```python
from build123d import *

# Parameters (mm, degrees)
SKETCH1_W           = 101.6
SKETCH1_H           = 76.2
BOSS_EXTRUDE1_DEPTH = 38.1
SKETCH3_W           = 97.6
SKETCH3_H           = 72.2
CUT_EXTRUDE1_DEPTH  = 36.1
SKETCH7_R           = 2.54
CUT_EXTRUDE2_DEPTH  = 2
SKETCH9_R           = 4
CUT_EXTRUDE3_DEPTH  = 2
SKETCH11_R          = 3.175
CUT_EXTRUDE4_DEPTH  = 2
FILLET1_R           = 5
FILLET2_R           = 5
CUT_EXTRUDE5_DEPTH  = 1


with BuildPart() as part:
    # Sketch1 → Boss-Extrude1 (new body)
    with BuildSketch(Plane(origin=(0, 0, 0), x_dir=(1, 0, 0), z_dir=(0, 1, 0))):
        Rectangle(SKETCH1_W, SKETCH1_H)
    extrude(amount=BOSS_EXTRUDE1_DEPTH)

    # Sketch3 → Cut-Extrude1 (cut)
    with BuildSketch(Plane(origin=(0, 38.1, 0), x_dir=(1, 0, 0), z_dir=(0, 1, 0))):
        Rectangle(SKETCH3_W, SKETCH3_H)
    extrude(amount=-CUT_EXTRUDE1_DEPTH, mode=Mode.SUBTRACT)

    # Sketch7 → Cut-Extrude2 (cut)
    with BuildSketch(Plane(origin=(50.8, 0, 0), x_dir=(0, 0, -1), z_dir=(1, 0, 0))):
        with Locations((-19.05, 19.05)):
            Circle(SKETCH7_R)
        with Locations((19.05, 19.05)):
            Circle(SKETCH7_R)
    extrude(amount=-CUT_EXTRUDE2_DEPTH, mode=Mode.SUBTRACT)

    # Sketch9 → Cut-Extrude3 (cut)
    with BuildSketch(Plane.ZY.offset(50.8)):
        with Locations((0, 19.05)):
            Circle(SKETCH9_R)
    extrude(amount=-CUT_EXTRUDE3_DEPTH, mode=Mode.SUBTRACT)

    # Sketch11 → Cut-Extrude4 (cut)
    with BuildSketch(Plane.XY.offset(38.1)):
        with Locations((-34.127797524, 19.05)):
            Circle(SKETCH11_R)
    extrude(amount=-CUT_EXTRUDE4_DEPTH, mode=Mode.SUBTRACT)

    # Fillet1
    fillet1_edges = [part.edges().sort_by_distance(p)[0] for p in [
        (50.8, 19.05, 38.1),
        (-50.8, 19.05, 38.1),
        (-50.8, 19.05, -38.1),
        (50.8, 19.05, -38.1),
    ]]
    fillet(fillet1_edges, radius=FILLET1_R)

    # Fillet2
    fillet2_edges = [part.edges().sort_by_distance(p)[0] for p in [
        (48.8, 20.05, 36.1),
        (-48.8, 20.05, 36.1),
        (-48.8, 20.05, -36.1),
        (48.8, 20.05, -36.1),
    ]]
    fillet(fillet2_edges, radius=FILLET2_R)

    # Sketch12 → Cut-Extrude5 (cut)
    # profile 1 of 2: a face of its own
    with BuildSketch(Plane.XZ):
        Polygon((-16.893847177, 6.052120704), (-32.260033074, 6.052120704), (-24.77410559, 22.334171986), (-24.386134837, 22.334171986), align=None)
        Polygon((-19.09446817, 7.476800191), (-24.576940125, 19.395770544), (-30.056231992, 7.476800191), align=None, mode=Mode.SUBTRACT)
    # profile 2 of 2: a face of its own
    with BuildSketch(Plane.XZ):
        Polygon((-6.564920895, 6.052120704), (-15.774456151, 6.052120704), (-11.338233194, 14.110464053), (-15.774456151, 21.927120704), (-6.768446536, 21.927120704), (-6.768446536, 20.298915576), (-13.255826343, 20.298915576), (-9.61780551, 13.887857884), (-13.144523258, 7.476800191), (-6.564920895, 7.476800191), align=None)
    extrude(amount=-CUT_EXTRUDE5_DEPTH, mode=Mode.SUBTRACT)


solid = part.part
```
Read the model definition and answer for the solid it produces. Units are mm, in the model's axes. A direction names the side the tool comes from. Round coordinates to 2 decimals unless told otherwise and drop trailing zeros. Write each loop counter-clockwise with the first axis right and the second up, starting at its lowest first coordinate (ties: lowest second). Pieces come first, ordered by that corner, then holes. Notation, with made-up numbers: M 81,27.5 L 108,27.5 A34 ccw 108,66.5 Z; hole C 54,-34 d8. An arc over 180 degrees is marked long. One line per item, written item: value.
Q1. Find section A-A on z = 0. Write down the section's boundary in (x, y).
Data:
outline: M -50.8,0 L 50.8,0 L 50.8,38.1 L 48.8,38.1 L 48.8,2 L -48.8,2 L -48.8,15.05 L -50.8,15.05 Z; M -50.8,23.05 L -48.8,23.05 L -48.8,38.1 L -50.8,38.1 Z
Q2. Flat-ended cylindrical pins translate along their axes: pin 1 Ø10 at (x, z) = (7.5, -10.5) entering from +Y; pin 2 Ø4 at (y, z) = (20, -1.5) entering from -X; pin 3 Ø1.5 at (x, z) = (12, -25) entering from -Y. Find the tip coordinate at first contact, or state that the pin passes through.
Data:
pin 1: y = 2
pin 2: x = 48.8
pin 3: y = 0
Q3. Which of the six approach directions +Z, -Z, +X, -X, +Y, -Y give full straight-line access (tool end or side, diameter ignored) to faces 1 (the flat face through (-1, 19, 38.1)), 2 (the cylindrical face through (-49.37, 19.32, -36.6)), 3 (the cylindrical face through (-49.814, 15.145, -0.867)), 4 (the flat face through (-27.28, 0.49, 13.52)), 5 (the flat face through (-48.8, 24, 0))?
Data:
face 1: +Z, +X, -X, +Y, -Y
face 2: -Z, -X, +Y, -Y
face 3: -X
face 4: -Y
face 5: +Y
Q4. For a pull along Y with two mould halves and no side action, classify faces 6 (the flat face through (-1, 0, -1)), 7 (the flat face through (-11.356, 0.493, 10.727)), 8 (the cylindrical face through (49.81, 16.57, -18.5)) as +Y half, -Y half, draft (parallel to the pull), parting line (faces both ways), or undercut.
Data:
face 6: -Y half
face 7: draft
face 8: undercut
Q5. Find section B-B on y = 12. Write down the section's boundary in (x, z), plus the area to 3 significant figures.
Data:
outline: M -50.8,-33.1 A5 ccw -45.8,-38.1 L 45.8,-38.1 A5 ccw 50.8,-33.1 L 50.8,33.1 A5 ccw 45.8,38.1 L -45.8,38.1 A5 ccw -50.8,33.1 Z; hole M -48.8,-31.1 A5 ccw -43.8,-36.1 L 43.8,-36.1 A5 ccw 48.8,-31.1 L 48.8,31.1 A5 ccw 43.8,36.1 L -43.8,36.1 A5 ccw -48.8,31.1 Z
area: 695 mm2
Q6. Find section C-C on y = 19.05. Count the separate pieces of the cut face and the enclosed holes in it, plus the area to 3 significant figures.
Data:
separate pieces: 4
enclosed holes: 0
area: 646 mm2
Q7. Find section D-D on x = 29. Write down the section's boundary in (y, z).
Data:
outline: M 0,-38.1 L 38.1,-38.1 L 38.1,-36.1 L 2,-36.1 L 2,36.1 L 38.1,36.1 L 38.1,38.1 L 0,38.1 Z
Q8. Straight lines are drawn through the part: line 1 (Y direction, x = 49.6, z = 19.05); line 2 (Z direction, x = 40, y = 27.5); line 3 (X direction, y = 33, z = -14). For each, find the intervals that lie inside material, in ascending order. Write a range as [from, to].
Data:
line 1: [0, 16.51], [21.59, 38.1]
line 2: [-38.1, -36.1], [36.1, 38.1]
line 3: [-50.8, -48.8], [48.8, 50.8]
